Input: part model. Units: mm. Frame: model coordinates. Face numbers are marked on the shaded views. A direction names the side the tool comes from. Round coordinates to 2 decimals unless told otherwise and drop trailing zeros. Write each loop counter-clockwise with the first axis right and the second up, starting at its lowest first coordinate (ties: lowest second). Pieces come first, ordered by that corner, then holes. Notation, with made-up numbers: M -32.75,34.25 L -25.75,34.25 A19 cw -25.75,60.25 Z; hole C -20.75,72.25 d8. An arc over 180 degrees is marked long. Write each question's results on one line, items separated by ' | '. Start each with the question number.
```python
from build123d import *

# Parameters (mm, degrees)
SKETCH3_W           = 20
SKETCH3_H           = 70
BOSS_EXTRUDE3_DEPTH = 5
CUT_EXTRUDE2_DEPTH  = 2
SKETCH6_R           = 3.57
CUT_EXTRUDE3_DEPTH  = 3
SKETCH7_R           = 1.175
SKETCH7_W           = 12.35
SKETCH7_H           = 23
CUT_EXTRUDE4_DEPTH  = 5
SKETCH8_W           = 1.25
SKETCH8_H           = 25
CUT_EXTRUDE5_DEPTH  = 30


with BuildPart() as part:
    # Sketch3 → Boss-Extrude3 (new body)
    with BuildSketch(Plane.XY):
        Rectangle(SKETCH3_W, SKETCH3_H)
    extrude(amount=BOSS_EXTRUDE3_DEPTH)

    # Sketch4 → Cut-Extrude2 (cut)
    with BuildSketch(Plane.XY.offset(5)):
        with BuildLine():
            Line((-2.85, 24.850023256), (-1.875, 12.739206809))
            Line((-1.875, 12.739206809), (1.875, 12.739206809))
            Line((1.875, 12.739206809), (2.85, 24.850023256))
            ThreePointArc((2.85, 24.850023256), (0, 23.43), (-2.85, 24.850023256))
        make_face()
        with BuildLine():
            Line((1.875, 12.739206809), (-1.875, 12.739206809))
            ThreePointArc((-1.875, 12.739206809), (0, 10.864206809), (1.875, 12.739206809))
        make_face()
        with BuildLine():
            ThreePointArc((3.57, 27), (-1.133666618, 30.385217866), (-2.85, 24.850023256))
            Line((-2.85, 24.850023256), (2.85, 24.850023256))
            ThreePointArc((2.85, 24.850023256), (3.385217866, 25.866333382), (3.57, 27))
        make_face()
        with BuildLine():
            Line((2.85, 24.850023256), (-2.85, 24.850023256))
            ThreePointArc((-2.85, 24.850023256), (0, 23.43), (2.85, 24.850023256))
        make_face()
    extrude(amount=-CUT_EXTRUDE2_DEPTH, mode=Mode.SUBTRACT)

    # Sketch6 → Cut-Extrude3 (cut)
    with BuildSketch(Plane.XY.offset(3)):
        with Locations((0, 27)):
            Circle(SKETCH6_R)
    extrude(amount=-CUT_EXTRUDE3_DEPTH, mode=Mode.SUBTRACT)

    # Sketch7 → Cut-Extrude4 (cut)
    with BuildSketch(Plane.XY.offset(5)):
        with Locations((0, -4.18)):
            Circle(SKETCH7_R)
        with Locations((0, -31.82)):
            Circle(SKETCH7_R)
        with Locations((0, -18)):
            Rectangle(SKETCH7_W, SKETCH7_H)
    extrude(amount=-CUT_EXTRUDE4_DEPTH, mode=Mode.SUBTRACT)

    # Sketch8 → Cut-Extrude5 (cut)
    with BuildSketch(Plane(origin=(10, 0, 0), x_dir=(0, 0, -1), z_dir=(1, 0, 0))):
        with Locations((-0.625, 22.5)):
            Rectangle(SKETCH8_W, SKETCH8_H)
    extrude(amount=-CUT_EXTRUDE5_DEPTH, mode=Mode.SUBTRACT)


solid = part.part
```
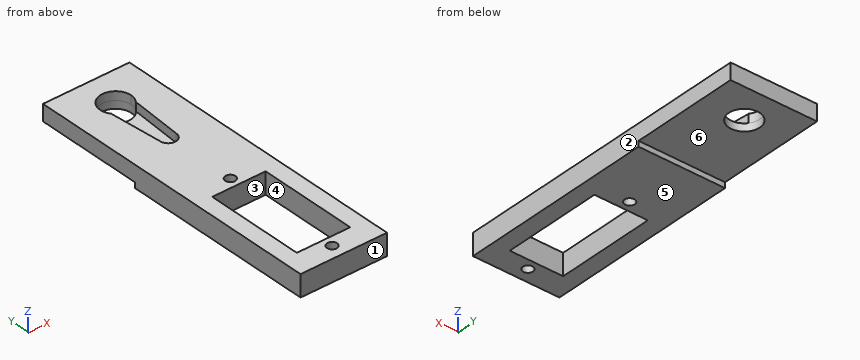
1. Cut plane C-C on z = 0.6. Output: boundary loops of the cut face in (x, y) (3 decimals), and give its area (3 significant figures).
2. Cut plane A-A on x = 0. Output: boundary loops of the cut face in (y, z) (3 decimals), and give its area (3 significant figures).
3. Access query for the marked faces 4, 5 and 6. Directions: +Z, -Z, +X, -X, +Y, -Y. A direction counts if a zero-diameter tool reaches every point of the face in a straight line with its end or side. Return the directions, or none.
4. Contact query for flat-ended pins moving along their axis: P1, Ø9.5, axis at x = 0, y = 27, coming from the -Z side; P2, Ø0.6, axis at x = -4, z = 0.5, coming from the +Y side; P3, Ø6.5, axis at x = 0, y = 27, coming from the -Z side; P4, Ø1.7, axis at x = -0.5, y = 20.5, coming from the +Z side. Output: stop coordinate, or through.
5. Draft query along Y for the marked faces 1, 2 and 3. Return one class per face: +Y half, -Y half, draft (parallel to the pull), parting line (faces both ways), or undercut.
6. Line query: L1, parallel to Y at x = 0, z = 2.4 (3 decimals); L2, parallel to Y at x = 0, z = 3.45 (3 decimals); L3, parallel to X at y = -9, z = 4.15 (3 decimals). Output: solid intervals per line, ascending. Write a range as from..to.
7. Cut plane B-B on y = -4.18. Output: boundary loops of the cut face in (x, z) (3 decimals).
8. Cut plane D-D on z = 4.4. Output: boundary loops of the cut face in (x, y) (3 decimals), and give its area (3 significant figures).
Answers follow:
1) outline: M -10,-35 L 10,-35 L 10,10 L -10,10 Z; hole M -6.175,-29.5 L 6.175,-29.5 L 6.175,-6.5 L -6.175,-6.5 Z; hole C 0,-31.82 d2.35; hole C 0,-4.18 d2.35 | area: 607 mm2
2) outline: M -35,0 L -32.995,0 L -32.995,5 L -35,5 Z; M -30.645,0 L -29.5,0 L -29.5,5 L -30.645,5 Z; M -6.5,0 L -5.355,0 L -5.355,5 L -6.5,5 Z; M -3.005,0 L 10,0 L 10,1.25 L 23.43,1.25 L 23.43,3 L 10.864,3 L 10.864,5 L -3.005,5 Z; M 30.57,1.25 L 35,1.25 L 35,5 L 30.57,5 Z | area: 128 mm2
3) face 4: +Z, -Z | face 5: -Z, +X, -X, +Y, -Y | face 6: -Z, +X, -X, +Y
4) P1: stops at z = 1.25 | P2: stops at y = 10 | P3: passes through | P4: stops at z = 3
5) face 1: -Y half | face 2: draft | face 3: undercut
6) L1: y = -35..-32.995, -30.645..-29.5, -6.5..-5.355, -3.005..23.43, 30.57..35 | L2: y = -35..-32.995, -30.645..-29.5, -6.5..-5.355, -3.005..10.864, 30.57..35 | L3: x = -10..-6.175, 6.175..10
7) outline: M -10,0 L -1.175,0 L -1.175,5 L -10,5 Z; M 1.175,0 L 10,0 L 10,5 L 1.175,5 Z
8) outline: M -10,-35 L 10,-35 L 10,35 L -10,35 Z; hole M -6.175,-29.5 L 6.175,-29.5 L 6.175,-6.5 L -6.175,-6.5 Z; hole M -2.85,24.85 L -1.875,12.739 A1.875 ccw 1.875,12.739 L 2.85,24.85 A3.57 ccw long Z; hole C 0,-31.82 d2.35; hole C 0,-4.18 d2.35 | area: 1,010 mm2
